Autodesk Inventor part; units mm, degrees
ref_plane "YZ Plane" through (0, 0, 0) normal (1, 0, 0) x (0, 1, 0)
ref_plane "XZ Plane" through (0, 0, 0) normal (0, 1, 0) x (-1, 0, 0)
ref_plane "XY Plane" through (0, 0, 0) normal (0, 0, 1) x (1, 0, 0)
sketch "Esboço1" plane through (0, 0, 0) normal (0, 0, 1) x (1, 0, 0)
  line L0 (-11.5, 5) -> (11.5, 5)
  line L1 (11.5, 5) -> (11.5, -5)
  line L2 (11.5, -5) -> (-11.5, -5)
  line L3 (-11.5, -5) -> (-11.5, 5)
  line L4 (-11.5, 5) -> (11.5, -5) construction
  line L5 (11.5, 5) -> (-11.5, -5) construction
  point P0 (0, 0)
  dimension "d0" = 10
  dimension "d1" = 23
extrude "Extrusão1" add sketch "Esboço1" along normal blind 15
chamfer "Chanfro1" distance 2 angle 45 2 edges at (-11.5, 0, 0) (11.5, 0, 0)
sketch "Esboço4" plane through (-11.5, -5, 15) normal (0, -1, 0) x (1, 0, 0)
  line L0 (11.5, -15) -> (11.5, -9)
  line L1 (3, -9) -> (20, -9) construction
  line L2 (3, -11) -> (20, -11)
  line L3 (20, -7) -> (3, -7)
  arc A0 (3, -7) -> (3, -11) centre (3, -9) ccw
  arc A1 (20, -11) -> (20, -7) centre (20, -9) ccw
  line L4 (23, -13) -> (23, 0)
  dimension "d18" = 6
  dimension "d19" = 4
  dimension "d20" = 3
extrude "Extrusão3" cut sketch "Esboço4" against normal through all
sketch "Esboço2" plane through (0, 0, 15) normal (0, 0, 1) x (1, 0, 0)
  line L0 (11.5, 5) -> (-11.5, 5)
  line L1 (-11.5, -5) -> (11.5, -5)
  line L2 (-9, -2.5) -> (9, -2.5)
  line L3 (0, 0) -> (0, -2.5)
  line L4 (-11.5, 5) -> (-11.5, -5)
  dimension "d32" = 2.5
  dimension "d36" = 2.5
hole "Furo1" at (-9, -2.5, 15) at (9, -2.5, 15) direction (0, 0, -1) diameter 2.459 depth 7.5 tip angle 118
sketch "Esboço5" plane through (0, 0, 0) normal (1, 0, 0) x (0, 1, 0)
  line L0 (5, 0) -> (-5, 0)
  line L1 (5, 0) -> (0, 0)
  line L2 (0, 0) -> (0, 12)
  line L3 (0, 12) -> (5, 12)
  line L4 (5, 12) -> (5, 0)
  line L5 (-5, 0) -> (-5, 2)
  line L6 (5, 15) -> (-5, 15)
  point P0 (0, 0)
  point P1 (2.5, 0)
  dimension "d27" = 5
  dimension "d29" = 3
extrude "Extrusão4" cut sketch "Esboço5" along normal through all both and the other way through all
chamfer "Chanfro2" distance 2.5 angle 45 1 edges at (0, 5, 12)
properties part number "SUPORTE ADAPTADOR USB TIPO C REV03 - PARTE 02" material "Alumínio 6061"
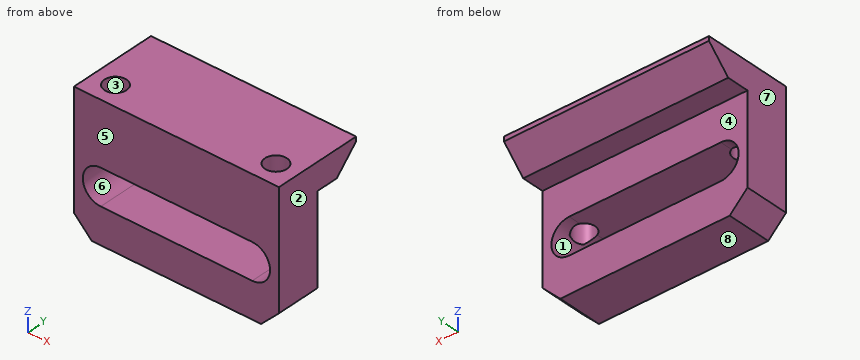
The model under review builds one solid part; all positions refer to its coordinate system, in mm. Face numbers are marked on the shaded views. A direction names the side the tool comes from. Give positions to 0.01 mm unless a question says otherwise; leave off trailing zeros. Order: outer loops, then holes, each group sorted by start corner. A loop starts at its lowest first (then second) coordinate and runs counter-clockwise, first axis right, second up. Notation, with made-up numbers: M 37.25,10.5 L 52.25,10.5 A11 cw 52.25,19.5 Z; hole C 82.25,-0.5 d8. An arc over 180 degrees is marked long. Use one line per item in the form item = value. Start each with the question number.
Item 1: We need section B-B on z = 14. Give the boundary of the cut face in (x, y).
Item 2: We need section D-D on y = -2.5. Give the boundary of the cut face in (x, z), plus the area to 3 significant figures.
Item 3: The part is to be moulded in two halves that separate along X. For the marked faces 6, 7 and 8, say which applies: pulls with the +X half, pulls with the -X half, needs draft (parallel to the pull), parting line crosses it, or undercut.
Item 4: We need section A-A on x = -3. Give the boundary of the cut face in (y, z), plus the area to 3 significant figures.
Item 5: To check wall thickness, follow line 1 along X through (y, z) = (-2.5, 12.5); line 2 along Z through (x, y) = (-1.5, -2); line 3 along Y through (x, z) = (9, 10.5). State the ranges of each line that lie inside material, in increasing order. Write a range as from..to.
Item 6: Insertion check: pin 1 Ø1.5 at (x, y) = (-1, -3) entering from -Z; pin 2 Ø6 at (y, z) = (3.5, 6.5) entering from +X; pin 3 Ø1 at (x, y) = (8, 2) entering from -Z. Each pin has a flat end and moves straight along its axis. Give the tip position at first contact, or say it passes through.
Item 7: For the marked faces 1, 2, 3, 4 and 5, list the 3-axis set-ups (+Z, -Z, +X, -X, +Y, -Y) from which the entire face can be reached by the end or side of a thin tool; tool diameter is ignored.
Item 8: We need section C-C on z = 5. Give the boundary of the cut face in (x, y).
Completed:
q1.outline = M -11.5,-5 L 11.5,-5 L 11.5,4.5 L -11.5,4.5 Z; hole C -9,-2.5 d2.46; hole C 9,-2.5 d2.46
q2.outline = M -11.5,2 L -9.5,0 L 9.5,0 L 11.5,2 L 11.5,15 L 10.23,15 L 10.23,7.5 L 9.98,7.35 A2 cw 8.5,4 L -8.5,4 A2 cw -9.98,7.35 L -10.23,7.5 L -10.23,15 L -11.5,15 Z; M -7.77,8 L 7.77,8 L 7.77,15 L -7.77,15 Z
q2.area = 225 mm²
q3.face_6 = undercut
q3.face_7 = pulls with the -X half
q3.face_8 = needs draft
q4.outline = M -5,0 L 0,0 L 0,4 L -5,4 Z; M -5,8 L 0,8 L 0,12 L 2.5,12 L 5,14.5 L 5,15 L -5,15 Z
q4.area = 66.9 mm²
q5.line_1 = -11.5..-10.23, -7.77..7.77, 10.23..11.5
q5.line_2 = 0..4, 8..15
q5.line_3 = -5..-3.73, -1.27..0
q6.pin_1 = 0
q6.pin_2 = through
q6.pin_3 = 12
q7.face_1 = +Y, -Y
q7.face_2 = +Z, -Z, +X, +Y, -Y
q7.face_3 = +Z
q7.face_4 = -Z, +X, -X, +Y
q7.face_5 = +Z, -Z, +X, -X, -Y
q8.outline = M -11.5,-5 L -10.23,-5 L -10.23,0 L -11.5,0 Z; M 10.23,-5 L 11.5,-5 L 11.5,0 L 10.23,0 Z
